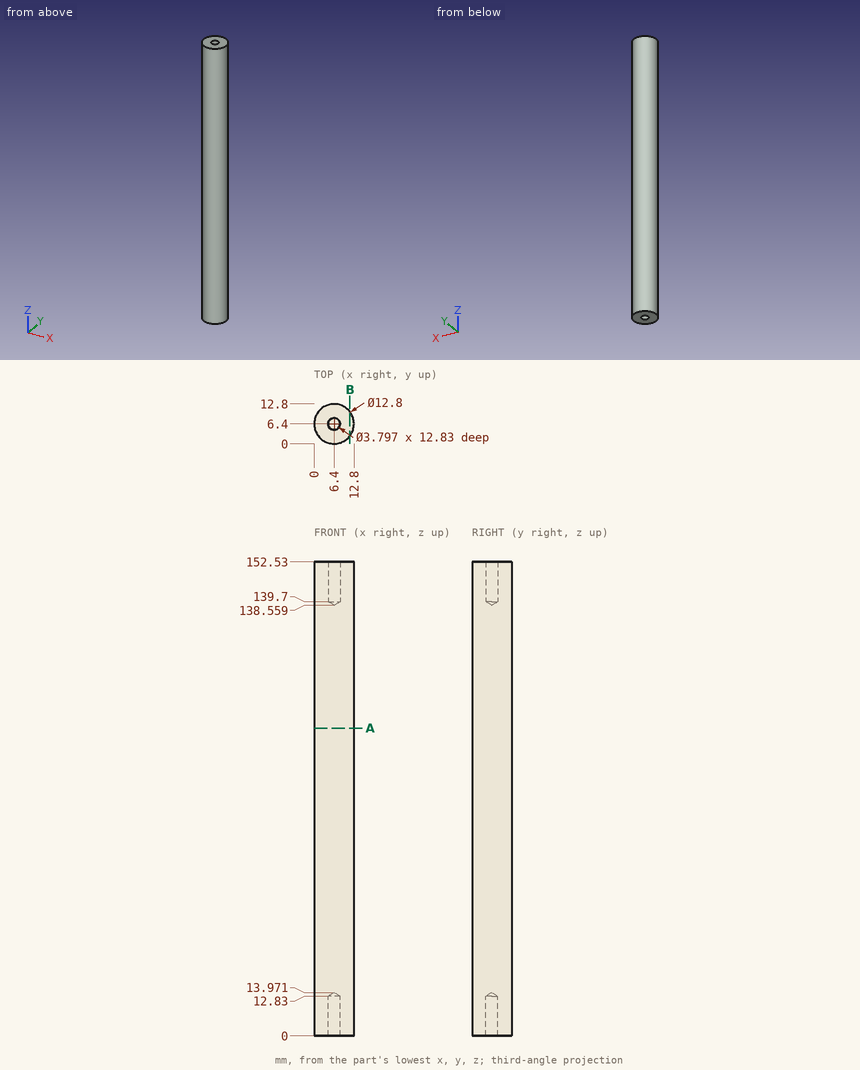
Here's the drawing with two shaded views (mm, measured from the low corner). I have some questions. Round coordinates to 2 decimals unless told otherwise and drop trailing zeros. Loops run counter-clockwise (first coordinate to the right, second up) from the corner with the lowest first, then second, coordinate; pieces in that order, holes last.
1. Suppose I cut it at B-B, the plane x = 11.5. Please give me the cut outline in (y, z), and give its area (3 significant figures).
Answers:
outline: (2.53, 0) - (10.27, 0) - (10.27, 152.53) - (2.53, 152.53) - close
area: 1,180 mm2
2. Suppose I cut it at A-A, the plane z = 99. Please give me the cut outline in (x, y), and give its area (3 significant figures).
Answers:
outline: circle Ø12.8 at (6.4, 6.4)
area: 129 mm2
3. Will these pins go through, and if not, where does the flat tip stop? pin 1 (6 mm diameter, centred on x = 4, z = 25.5, fed in from -Y); pin 2 (3.5 mm diameter, centred on x = 6.4, y = 6.4, fed in from +Z); pin 3 (2 mm diameter, centred on y = 3.5, z = 26, fed in from +X); pin 4 (1.5 mm diameter, centred on x = 5.5, z = 24.5, fed in from +Y).
Answers:
pin 1: stops at y = 0
pin 2: stops at z = 139.61
pin 3: stops at x = 12.51
pin 4: stops at y = 12.8
4. If I drill on probe 1 along Y at (x, z) = (6, 39); probe 2 along Y at (x, z) = (6.4, 148); probe 3 along X at (y, z) = (6, 9), over which ranges is the centre line in solid material (lowest first)?
Answers:
probe 1: y = 0.01 to 12.79
probe 2: y = 0 to 4.5, 8.3 to 12.8
probe 3: x = 0.01 to 4.54, 8.26 to 12.79
